Geometry check sheet. Reference: drawing and pictorial views, mm from the part's lowest x, y, z. Coordinates: 2 decimals unless noted, no trailing zeros. Write each loop counter-clockwise with the first axis right and the second up, starting at its lowest first coordinate (ties: lowest second). Pieces come first, ordered by that corner, then holes. Notation, with made-up numbers: (79, 4.5) -> (136, 4.5) arc R16 cw to (136, 17.5) -> close; hole circle Ø2 at (60, 37). An arc over 180 degrees is marked (long way). Use a Markdown table: item, result.
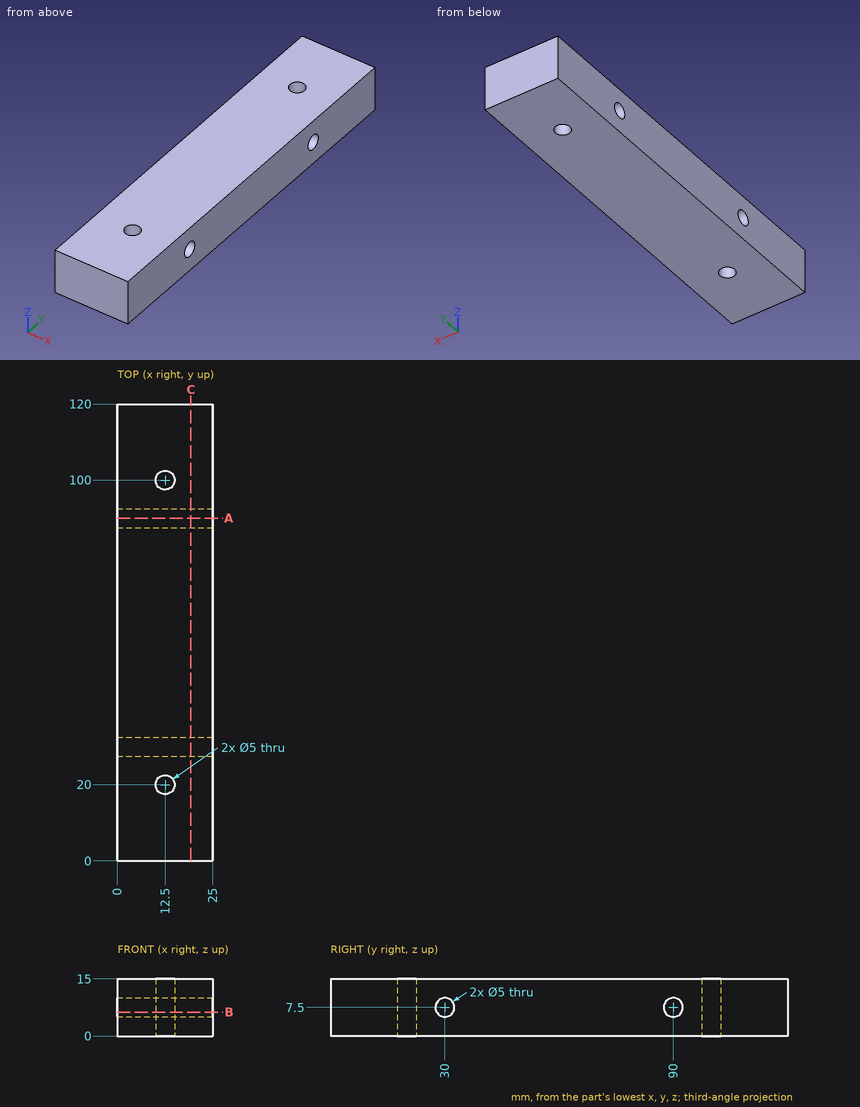
Item 1: Section check C-C on x = 19.25. Record the boundary of the cut face in (y, z).
Answer block:
| item | result |
|---|---|
| outline | (0, 0) -> (120, 0) -> (120, 15) -> (0, 15) -> close; hole circle Ø5 at (30, 7.5); hole circle Ø5 at (90, 7.5) |
Item 2: Thickness scan on L1, parallel to Y at x = 19.75, z = 7.5; L2, parallel to Y at x = 12.5, z = 12; L3, parallel to Y at x = 10.5, z = 7.5. Record the ranges inside material, lowest first. Write a range as [from, to].
Answer block:
| item | result |
|---|---|
| L1 | y = [0, 27.5], [32.5, 87.5], [92.5, 120] |
| L2 | y = [0, 17.5], [22.5, 97.5], [102.5, 120] |
| L3 | y = [0, 18.5], [21.5, 27.5], [32.5, 87.5], [92.5, 98.5], [101.5, 120] |
Item 3: Section check B-B on z = 6.25. Record the boundary of the cut face in (x, y), then the cut area to 3 significant figures.
Answer block:
| item | result |
|---|---|
| outline | (0, 0) -> (25, 0) -> (25, 27.83) -> (0, 27.83) -> close; (0, 32.17) -> (25, 32.17) -> (25, 87.83) -> (0, 87.83) -> close; (0, 92.17) -> (25, 92.17) -> (25, 120) -> (0, 120) -> close; hole circle Ø5 at (12.5, 20); hole circle Ø5 at (12.5, 100) |
| area | 2,740 mm^2 |
Item 4: Section check A-A on y = 90. Record the boundary of the cut face in (x, z).
Answer block:
| item | result |
|---|---|
| outline | (0, 0) -> (25, 0) -> (25, 5) -> (0, 5) -> close; (0, 10) -> (25, 10) -> (25, 15) -> (0, 15) -> close |
Item 5: Depth check by flat-ended pin: P1, Ø4, axis at y = 90, z = 7.5, coming from the +X side. Enter the tip coordinate at first touch or a pass-through.
Answer block:
| item | result |
|---|---|
| P1 | passes through |
